Source: CAD feature listing. Evaluate the final solid. Frame: model axes, mm. A direction names the side the tool comes from. Round coordinates to 2 decimals unless told otherwise and drop trailing zeros. Order: outer loops, then holes, each group sorted by start corner. A loop starts at its lowest first (then second) coordinate and runs counter-clockwise, first axis right, second up. Notation, with made-up numbers: (-2.75, -24.75) - (26.25, -24.75) arc R19 cw to (26.25, -16.75) - close; hole circle Ø3 at (69.25, -16.5). An arc over 180 degrees is marked (long way). Use one line per item in the form item = value. Start each with the question number.
Q1. Cut plane A-A, the plane z = 25.4. Return the cut outline in (x, y).
Q2. Pin query (flat end, axial travel): pin 1 Ø7.5 at (x, z) = (38.1, 63.5) entering from -Y; pin 2 Ø8 at (x, z) = (-53, 51.5) entering from +Y; pin 3 Ø19 at (y, z) = (27.5, 46.5) entering from -X. Return the tip coordinate at first contact, or that it passes through.
Q3. Cut plane B-B, the plane x = 38.1. Return the cut outline in (y, z), and give its area (3 significant figures).
Q4. Set-up query: faces 5 (the flat face through (-50, 15.039, 38)), 6 (the flat face through (25, 53.139, 38)). Return all of +Z, -Z, +X, -X, +Y, -Y with unobstructed straight access to the full face (end or side cutting, diameter ignored); none if empty.
Q5. Cut plane C-C, the plane y = 27. Return the cut outline in (x, z).
Q6. Draft query along X for faces 1 (the cylindrical face through (32.234, 15.573, 22.968)), 2 (the cylindrical face through (39.48, 15.57, 57.3)), 3 (the flat face through (-1, -23.061, 38)), 4 (the flat face through (-76.2, -4, 38)). Return one class per face: released by +X, released by -X, zero draft, split by the parting line, or undercut.
Q7. Ray query, line 1 (Z direction, x = 38, y = 32); line 2 (X direction, y = 35, z = 25); line 3 (X direction, y = 8, z = 25.5). Return the intervals inside material, ascending. Write a range as [from, to].
Q8. Cut plane D-D, the plane z = 16. Return the cut outline in (x, y), and give its area (3 significant figures).
from build123d import *

# Parameters (mm, degrees)
F0_W     = 101.6
F0_H     = 38.1
F1_DEPTH = 76.2
F2_R     = 6.35
F3_DEPTH = 76.2


with BuildPart() as f1:
    # F0 (on Top) → F1 (new body)
    with BuildSketch(Plane.XY):
        Polygon((76.2, -23.060526), (76.2, 15.039474), (-25.4, 15.039474), (-76.2, 15.039474), (-76.2, -23.060526), align=None)
        with Locations((25.4, 34.089474)):
            Rectangle(F0_W, F0_H)
    extrude(amount=F1_DEPTH)

    # F2 (on face) → F3 (cut)
    with BuildSketch(Plane(origin=(0, 53.139474, 0), x_dir=(-1, 0, 0), z_dir=(0, 1, 0))):
        with Locations((-38.1, 25.4)):
            Circle(F2_R)
        with Locations((-38.1, 63.5)):
            Circle(F2_R)
    extrude(amount=-F3_DEPTH, mode=Mode.SUBTRACT)


solid = f1.part
Completed:
q1.outline = (-76.2, -23.06) - (31.75, -23.06) - (31.75, 53.14) - (-25.4, 53.14) - (-25.4, 15.04) - (-76.2, 15.04) - close; (44.45, -23.06) - (76.2, -23.06) - (76.2, 53.14) - (44.45, 53.14) - close
q2.pin_1 = through
q2.pin_2 = 15.04
q2.pin_3 = -25.4
q3.outline = (-23.06, 0) - (53.14, 0) - (53.14, 19.05) - (-23.06, 19.05) - close; (-23.06, 31.75) - (53.14, 31.75) - (53.14, 57.15) - (-23.06, 57.15) - close; (-23.06, 69.85) - (53.14, 69.85) - (53.14, 76.2) - (-23.06, 76.2) - close
q3.area = 3,870 mm2
q4.face_5 = +Z, -Z, -X, +Y
q4.face_6 = +Z, -Z, +X, -X, +Y
q5.outline = (-25.4, 0) - (76.2, 0) - (76.2, 76.2) - (-25.4, 76.2) - close; hole circle Ø12.7 at (38.1, 25.4); hole circle Ø12.7 at (38.1, 63.5)
q6.face_1 = undercut
q6.face_2 = undercut
q6.face_3 = zero draft
q6.face_4 = released by -X
q7.line_1 = [0, 19.05], [31.75, 57.15], [69.85, 76.2]
q7.line_2 = [-25.4, 31.76], [44.44, 76.2]
q7.line_3 = [-76.2, 31.75], [44.45, 76.2]
q8.outline = (-76.2, -23.06) - (76.2, -23.06) - (76.2, 53.14) - (-25.4, 53.14) - (-25.4, 15.04) - (-76.2, 15.04) - close
q8.area = 9,680 mm2
